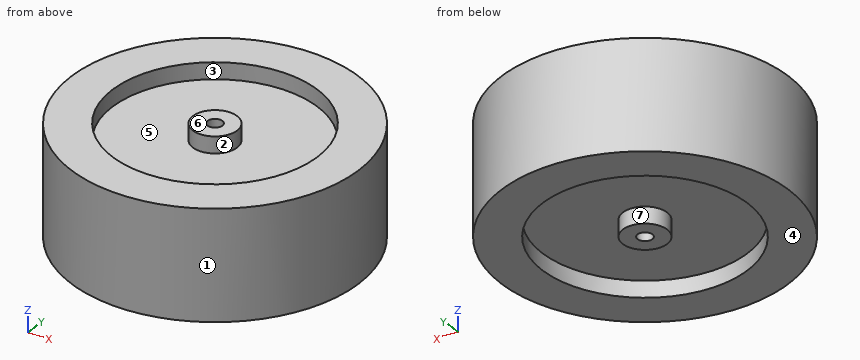
Autodesk Inventor part; units mm, degrees
ref_plane "Plano de trabalho1" through (0, 0, 13.3) normal (0, 0, 1) x (1, 0, 0)
ref_plane "YZ Plane" through (0, 0, 0) normal (1, 0, 0) x (0, 1, 0)
ref_plane "XZ Plane" through (0, 0, 0) normal (0, 1, 0) x (-1, 0, 0)
sketch "Esboço2" plane through (0, 0, 0) normal (0, 0, 1) x (1, 0, 0)
  circle A0 centre (0, 0) radius 35
  dimension "d5" = 70
extrude "Extrusão2" add sketch "Esboço2" along normal blind 26.6
sketch "Esboço9" plane through (0, 0, 26.6) normal (0, 0, 1) x (1, 0, 0)
  circle A0 centre (0, 0) radius 25
  dimension "d18" = 50
extrude "Extrusão5" cut sketch "Esboço9" against normal blind 4
sketch "Esboço12" plane through (0, 0, 22.6) normal (0, 0, 1) x (1, 0, 0)
  circle A0 centre (0, 0) radius 5.4
  dimension "d24" = 10.8
extrude "Extrusão7" add sketch "Esboço12" along normal blind 4
sketch "Esboço13" plane through (0, 0, 26.6) normal (0, 0, 1) x (1, 0, 0)
  circle A0 centre (0, 0) radius 1.8
  dimension "d27" = 3.6
extrude "Extrusão8" cut sketch "Esboço13" against normal through all
ref_plane "Plano de trabalho1" through (0, 0, 13.3) normal (0, 0, 1) x (1, 0, 0)
mirror "Espelhamento2" about plane through (0, 0, 13.3) normal (0, 0, 1) of "Extrusão8", "Extrusão7", "Extrusão5"
properties part number "roda"
The model under review builds one solid part; all positions refer to its coordinate system, in mm. Face numbers are marked on the shaded views. A direction names the side the tool comes from. Give positions to 0.01 mm unless a question says otherwise; leave off trailing zeros. Loops run counter-clockwise (first coordinate to the right, second up) from the corner with the lowest first, then second, coordinate; pieces in that order, holes last. Notation, with made-up numbers: (67, 85.5) -> (126, 85.5) arc R17 ccw to (126, 99.5) -> close; hole circle Ø8 at (25, 74). An arc over 180 degrees is marked (long way). Write each question's results on one line, items separated by ' | '.
1) Tool access review of the marked faces 5, 6 and 7: name each direction out of +Z, -Z, +X, -X, +Y, -Y from which nothing blocks a thin tool from reaching the whole face with its end or side.
Conclusion:
face 5: +Z | face 6: +Z, +X, -X, +Y, -Y | face 7: -Z
2) Insertion check: pin 1 Ø6 at (y, z) = (-28, 21) entering from +X; pin 2 Ø1 at (y, z) = (27, 12) entering from -X; pin 3 Ø1 at (y, z) = (18, 9.5) entering from +X; pin 4 Ø3 at (x, y) = (0, 0) entering from -Z. Each pin has a flat end and moves straight along its axis. Give the tip position at first contact, or say it passes through.
Conclusion:
pin 1: stops at x = 24.49 | pin 2: stops at x = -22.86 | pin 3: stops at x = 30.31 | pin 4: passes through
3) Take a section at A-A, the plane x = 0. Give the boundary of the cut face in (y, z), plus the area to 3 significant figures.
Conclusion:
outline: (-35, 0) -> (-25, 0) -> (-25, 4) -> (-5.4, 4) -> (-5.4, 0) -> (-1.8, 0) -> (-1.8, 26.6) -> (-5.4, 26.6) -> (-5.4, 22.6) -> (-25, 22.6) -> (-25, 26.6) -> (-35, 26.6) -> close; (1.8, 0) -> (5.4, 0) -> (5.4, 4) -> (25, 4) -> (25, 0) -> (35, 0) -> (35, 26.6) -> (25, 26.6) -> (25, 22.6) -> (5.4, 22.6) -> (5.4, 26.6) -> (1.8, 26.6) -> close | area: 1,450 mm^2
4) Take a section at C-C, the plane z = 16.75. Give the boundary of the cut face in (x, y), plus the area to 3 significant figures.
Conclusion:
outline: circle Ø70 at (0, 0); hole circle Ø3.6 at (0, 0) | area: 3,840 mm^2
5) Take a section at D-D, the plane x = 13. Give the boundary of the cut face in (y, z).
Conclusion:
outline: (-32.5, 0) -> (-21.35, 0) -> (-21.35, 4) -> (21.35, 4) -> (21.35, 0) -> (32.5, 0) -> (32.5, 26.6) -> (21.35, 26.6) -> (21.35, 22.6) -> (-21.35, 22.6) -> (-21.35, 26.6) -> (-32.5, 26.6) -> close
6) For line 1 along Y through (x, z) = (0, 1.15); line 2 along Y through (x, z) = (0, 11); line 3 along Z through (x, y) = (-14.5, -8.5), list the stretches that pass through material, from the lowest coordinate up. Write a range as from..to.
Conclusion:
line 1: y = -35..-25, -5.4..-1.8, 1.8..5.4, 25..35 | line 2: y = -35..-1.8, 1.8..35 | line 3: z = 4..22.6
7) Draft analysis for pull direction X (two halves, no side actions). For the marked faces 1, 2, 3 and 4, state which applies: pulls with the +X half, pulls with the -X half, needs draft (parallel to the pull), parting line crosses it, or undercut.
Conclusion:
face 1: parting line crosses it | face 2: undercut | face 3: undercut | face 4: needs draft
